Geometry check sheet. Reference: the model listing, model coordinates, mm. Round coordinates to 2 decimals unless told otherwise and drop trailing zeros. Write each loop counter-clockwise with the first axis right and the second up, starting at its lowest first coordinate (ties: lowest second). Pieces come first, ordered by that corner, then holes.
Item 1: Scan lines: probe 1 along Z at (x, y) = (-41, 1.5); probe 2 along Z at (x, y) = (-8.9, 2.35); probe 3 along Z at (x, y) = (-0.5, 2.3). Record each from-to range of solid material in increasing order.
Item 2: Cross-section at B-B (z = 0). State how many separate pieces and enclosed holes the cut face has, then the cut area to 3 significant figures.
Item 3: Cross-section at D-D (x = 49.4). Enter the section's corners in (y, z), then the cut area to 3 significant figures.
Item 4: Cross-section at A-A (x = 0). Enter the section's corners in (y, z).
Item 5: Depth check by flat-ended pin: P1, Ø10.5, axis at x = 41, z = 0, coming from the -Y side; P2, Ø3.5, axis at x = -8.9, z = 6.5, coming from the -Y side; P3, Ø1, axis at y = 1, z = -1.5, coming from the +X side; P4, Ø1.5, axis at y = 1.5, z = 8, coming from the -X side. Enter the tip coordinate at first touch or a pass-through.
from build123d import *

# Parameters (mm, degrees)
SKETCH1_R           = 4.5
SKETCH1_R_2         = 1.5
SKETCH1_R_3         = 3
BOSS_EXTRUDE1_DEPTH = 3.3


with BuildPart() as part:
    # Sketch1 → Boss-Extrude1 (new body)
    with BuildSketch(Plane(origin=(0, 0, 0), x_dir=(1, 0, 0), z_dir=(0, 1, 0))):
        with BuildLine():
            Line((41, -12), (-41, -12))
            ThreePointArc((-41, -12), (-53, 0), (-41, 12))
            Line((-41, 12), (41, 12))
            ThreePointArc((41, 12), (53, 0), (41, -12))
        make_face()
        with Locations((41, 0)):
            Circle(SKETCH1_R, mode=Mode.SUBTRACT)
        with Locations((41, 8.4)):
            Circle(SKETCH1_R_2, mode=Mode.SUBTRACT)
        with Locations((49.4, 0)):
            Circle(SKETCH1_R_2, mode=Mode.SUBTRACT)
        with Locations((41, -8.4)):
            Circle(SKETCH1_R_2, mode=Mode.SUBTRACT)
        with Locations((-41, -8.4)):
            Circle(SKETCH1_R_2, mode=Mode.SUBTRACT)
        with Locations((-49.4, 0)):
            Circle(SKETCH1_R_2, mode=Mode.SUBTRACT)
        with Locations((-41, 8.4)):
            Circle(SKETCH1_R_2, mode=Mode.SUBTRACT)
        with Locations((-41, 0)):
            Circle(SKETCH1_R, mode=Mode.SUBTRACT)
        with Locations((-8.9, 0)):
            Circle(SKETCH1_R_2, mode=Mode.SUBTRACT)
        with Locations((-8.9, 6.5)):
            Circle(SKETCH1_R_3, mode=Mode.SUBTRACT)
        with Locations((-8.9, -6.5)):
            Circle(SKETCH1_R_3, mode=Mode.SUBTRACT)
        with BuildLine():
            Line((-0.9, 8), (29.1, 8))
            ThreePointArc((29.1, 8), (31.221320344, 7.121320344), (32.1, 5))
            Line((32.1, 5), (32.1, -5))
            ThreePointArc((32.1, -5), (31.221320344, -7.121320344), (29.1, -8))
            Line((29.1, -8), (-0.9, -8))
            ThreePointArc((-0.9, -8), (-3.021320344, -7.121320344), (-3.9, -5))
            Line((-3.9, -5), (-3.9, 5))
            ThreePointArc((-3.9, 5), (-3.021320344, 7.121320344), (-0.9, 8))
        make_face(mode=Mode.SUBTRACT)
        with BuildLine():
            Line((-28.9, 8), (-16.9, 8))
            ThreePointArc((-16.9, 8), (-14.778679656, 7.121320344), (-13.9, 5))
            Line((-13.9, 5), (-13.9, -5))
            ThreePointArc((-13.9, -5), (-14.778679656, -7.121320344), (-16.9, -8))
            Line((-16.9, -8), (-28.9, -8))
            ThreePointArc((-28.9, -8), (-31.021320344, -7.121320344), (-31.9, -5))
            Line((-31.9, -5), (-31.9, 5))
            ThreePointArc((-31.9, 5), (-31.021320344, 7.121320344), (-28.9, 8))
        make_face(mode=Mode.SUBTRACT)
    extrude(amount=BOSS_EXTRUDE1_DEPTH)


solid = part.part
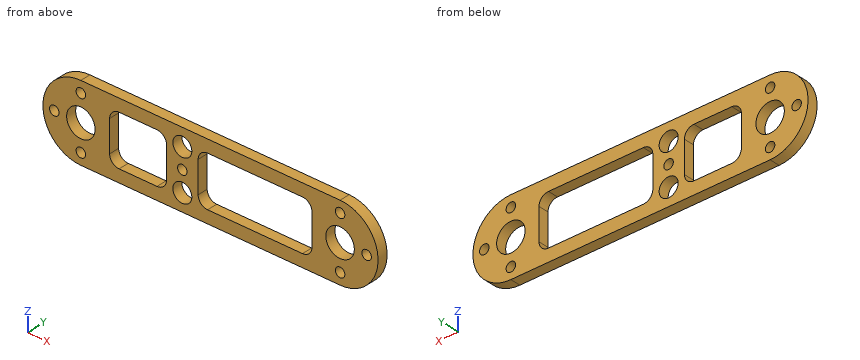
Resolved:
1. probe 1: z = -12 to -9.9, -6.9 to -4.5, 4.5 to 6.9, 9.9 to 12
1. probe 2: z = -12 to -9.5, -3.5 to -1.5, 1.5 to 3.5, 9.5 to 12
1. probe 3: z = -12 to -8, 8 to 12
2. separate pieces: 8
2. enclosed holes: 0
2. area: 82.5 mm2
3. outline: (0, -8.57) - (3.3, -8.57) - (3.3, -1.5) - (0, -1.5) - close; (0, 1.5) - (3.3, 1.5) - (3.3, 8.57) - (0, 8.57) - close
3. area: 46.7 mm2
4. outline: (0, -12) - (3.3, -12) - (3.3, -8) - (0, -8) - close; (0, 8) - (3.3, 8) - (3.3, 12) - (0, 12) - close
5. P1: stops at y = 0
5. P2: passes through
5. P3: stops at x = 52.96
5. P4: stops at x = -50.56
